Geometry check sheet. Reference: the model listing, model coordinates, mm. A direction names the side the tool comes from. Round coordinates to 2 decimals unless told otherwise and drop trailing zeros. Order: outer loops, then holes, each group sorted by start corner. A loop starts at its lowest first (then second) coordinate and runs counter-clockwise, first axis right, second up. Notation, with made-up numbers: (84.25, 54.5) - (134.25, 54.5) arc R18 ccw to (134.25, 62.5) - close; hole circle Ø9 at (-7, -29.75). An arc over 180 degrees is marked (long way). Use a Markdown table: item, result. Add a question column.
(1) Mould release check, pull along X, two halves, no side actions. Record for faces 4 (the face through (-22.9, 0, 2)), 5 (the face through (12, 34, 2)), 6 (the face through (5, -24, 3)): released by +X, released by -X, zero draft, split by the parting line, or undercut.
(2) Gauge pin test, flat ends, axial feed: P1, Ø8, axis at x = -4.5, y = 24, coming from the -Z side; P2, Ø1.5, axis at x = -1, z = 2.5, coming from the +Y side; P3, Ø2.5, axis at x = -0.5, z = 2, coming from the -Y side. Record the tip position at first contact, or that the pin passes through.
(3) Thickness scan on line 1 along X through (y, z) = (-28.5, 4.6); line 2 along Y through (x, z) = (-4.5, 3.75); line 3 along Y through (x, z) = (0.5, 4.45). Record the ranges inside material, lowest first. Write a range as [from, to].
(4) Section check A-A on y = 26. Record the boundary of the cut face in (x, z).
(5) Access from +Z, -Z, +X, -X, +Y, -Y to the whole of each face (thin tool, end or side, straight path). Record for faces 1 (the face through (-2.1, 31, 3)), 2 (the face through (5, 24, 3)), 3 (the face through (-2.1, -32, 3)).
(6) Section check B-B on z = 1.8. Record the boundary of the cut face in (x, y), then the cut area to 3 significant figures.
```python
from build123d import *

# Parameters (mm, degrees)
SKETCH1_W           = 45.8
SKETCH1_H           = 68
BOSS_EXTRUDE1_DEPTH = 5
CUT_EXTRUDE1_DEPTH  = 5


with BuildPart() as part:
    # Sketch1 → Boss-Extrude1 (new body)
    with BuildSketch(Plane.XY):
        Rectangle(SKETCH1_W, SKETCH1_H)
    extrude(amount=BOSS_EXTRUDE1_DEPTH)

    # Sketch2 → Cut-Extrude1 (cut)
    with BuildSketch(Plane.XY.offset(5)):
        Polygon((-2.1, 34), (2.1, 34), (2.1, 29), (5, 29), (5, 19), (-5, 19), (-5, 29), (-2.1, 29), align=None)
        Polygon((-2.1, -34), (-2.1, -29), (-5, -29), (-5, -19), (5, -19), (5, -29), (2.1, -29), (2.1, -34), align=None)
    extrude(amount=-CUT_EXTRUDE1_DEPTH, mode=Mode.SUBTRACT)


solid = part.part
```
Check sheet entries:
| question | item | result |
|---|---|---|
| 1 | face 4 | released by -X |
| 1 | face 5 | zero draft |
| 1 | face 6 | undercut |
| 2 | P1 | stops at z = 0 |
| 2 | P2 | stops at y = 19 |
| 2 | P3 | stops at y = -19 |
| 3 | line 1 | x = [-22.9, -5], [5, 22.9] |
| 3 | line 2 | y = [-34, -29], [-19, 19], [29, 34] |
| 3 | line 3 | y = [-19, 19] |
| 4 | outline | (-22.9, 0) - (-5, 0) - (-5, 5) - (-22.9, 5) - close; (5, 0) - (22.9, 0) - (22.9, 5) - (5, 5) - close |
| 5 | face 1 | +Z, -Z, +Y |
| 5 | face 2 | +Z, -Z |
| 5 | face 3 | +Z, -Z, -Y |
| 6 | outline | (-22.9, -34) - (-2.1, -34) - (-2.1, -29) - (-5, -29) - (-5, -19) - (5, -19) - (5, -29) - (2.1, -29) - (2.1, -34) - (22.9, -34) - (22.9, 34) - (2.1, 34) - (2.1, 29) - (5, 29) - (5, 19) - (-5, 19) - (-5, 29) - (-2.1, 29) - (-2.1, 34) - (-22.9, 34) - close |
| 6 | area | 2,870 mm2 |
